Autodesk Inventor part; units mm, degrees
ref_plane "YZ Plane" through (0, 0, 0) normal (1, 0, 0) x (0, 1, 0)
ref_plane "XZ Plane" through (0, 0, 0) normal (0, 1, 0) x (-1, 0, 0)
ref_plane "XY Plane" through (0, 0, 0) normal (0, 0, 1) x (1, 0, 0)
sketch "Skizze1" plane through (0, 0, 0) normal (1, 0, 0) x (0, 1, 0)
  line L0 (10, 115) -> (-10, 115)
  line L1 (-10, 115) -> (-10, -115)
  line L2 (-10, -115) -> (10, -115)
  line L3 (10, -115) -> (10, 115)
  line L4 (10, 115) -> (-10, -115) construction
  line L5 (-10, 115) -> (10, -115) construction
  point P0 (0, 0)
  dimension "d0" = 230
  dimension "d1" = 20
extrude "Extrusion1" add sketch "Skizze1" along normal blind 10
sketch "Skizze2" plane through (0, 0, 0) normal (-1, 0, 0) x (0, 0, 1)
  line L0 (-115, -10) -> (-115, 10)
  point P0 (0, 0)
  point P1 (-107, 0)
  point P2 (0, 0)
  point P3 (107, 0)
  dimension "d4" = 8
  dimension "d5" = 107
  dimension "d13" = 107
hole "Bohrung1" at (0, 0, -107) at (0, 0, 0) at (0, 0, 107) direction (1, 0, 0) diameter 4.5 end through all
fillet "Rundung1" radius 4 4 edges at (5, 10, -115) (5, -10, -115) (5, -10, 115) (5, 10, 115)
properties part number "103.018.01_Distanz_Wand"
Read the model definition and answer for the solid it produces. Units are mm, in the model's axes. Coordinates: 2 decimals unless noted, no trailing zeros. Loops run counter-clockwise (first coordinate to the right, second up) from the corner with the lowest first, then second, coordinate; pieces in that order, holes last. Notation, with made-up numbers: (47.25, 85) -> (102.25, 85) arc R10 cw to (102.25, 89) -> close; hole circle Ø2 at (-9, 44.25). An arc over 180 degrees is marked (long way). Return JSON: item names as keys, results as strings.
Item 1: Find section A-A (y = 0). Determine the outline of the cut face in (x, z).
Answers:
{"outline": "(0, -115) -> (10, -115) -> (10, -109.25) -> (0, -109.25) -> close; (0, -104.75) -> (10, -104.75) -> (10, -2.25) -> (0, -2.25) -> close; (0, 2.25) -> (10, 2.25) -> (10, 104.75) -> (0, 104.75) -> close; (0, 109.25) -> (10, 109.25) -> (10, 115) -> (0, 115) -> close"}
Item 2: Flat-ended cylindrical pins translate along their axes: P1, Ø5, axis at y = 0, z = 0, coming from the +X side; P2, Ø3.5, axis at y = 0, z = -107, coming from the +X side. Find the tip coordinate at first contact, or state that the pin passes through.
Answers:
{"P1": "stops at x = 10", "P2": "passes through"}
Item 3: Find section B-B (z = -107). Determine the outline of the cut face in (x, y), plus the area to 3 significant figures.
Answers:
{"outline": "(0, -10) -> (10, -10) -> (10, -2.25) -> (0, -2.25) -> close; (0, 2.25) -> (10, 2.25) -> (10, 10) -> (0, 10) -> close", "area": "155 mm2"}
Item 4: Find the intervals of material crossed by probe 1 along Z at (x, y) = (6, 0); probe 2 along Z at (x, y) = (5.25, -1.25); probe 3 along Y at (x, z) = (4, 0), in increasing order.
Answers:
{"probe 1": "z = -115 to -109.25, -104.75 to -2.25, 2.25 to 104.75, 109.25 to 115", "probe 2": "z = -115 to -108.87, -105.13 to -1.87, 1.87 to 105.13, 108.87 to 115", "probe 3": "y = -10 to -2.25, 2.25 to 10"}
Item 5: For a pull along Y with two mould halves and no side action, classify faces 1 (the cylindrical face through (5.07, -8.859, -113.797)), 2 (the cylindrical face through (5.07, 0.86, -104.92)), 3 (the flat face through (5, 0, 115)) as +Y half, -Y half, draft (parallel to the pull), parting line (faces both ways), or undercut.
Answers:
{"face 1": "-Y half", "face 2": "undercut", "face 3": "draft"}
